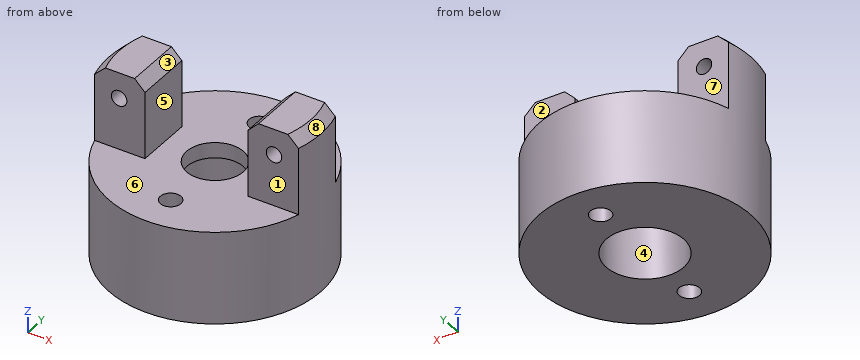
from build123d import *

# Parameters (mm, degrees)
SKETCH_1_R          = 20.5
EXTRUDE_1_DEPTH     = 33
CUT_EXTRUDE_1_DEPTH = 15
SKETCH_3_R          = 5
SKETCH_3_R_2        = 2
CUT_EXTRUDE_2_DEPTH = 35.124771062
CHAMFER_1_SIZE      = 2
SKETCH_4_R          = 1.5
CUT_EXTRUDE_3_DEPTH = 15
SKETCH_6_R          = 5.5
CUT_EXTRUDE_4_DEPTH = 35.124771062
SKETCH_9_R          = 7.5
CUT_EXTRUDE_7_DEPTH = 15


with BuildPart() as part:
    # Эскиз1 → Вытянуть1 (new body)
    with BuildSketch(Plane.XY):
        Circle(SKETCH_1_R)
    extrude(amount=EXTRUDE_1_DEPTH)

    # Эскиз2 → Вырез-Вытянуть1 (cut)
    with BuildSketch(Plane.XY.offset(33)):
        Polygon((10, 5.5), (24.402362137, 5.5), (24.402362137, 27.166317261), (-29.05675736, 27.166317261), (-29.05675736, 5.5), (-10, 5.5), (-10, -5.5), (-25.152295152, -5.5), (-25.152295152, -27.51572327), (25.537931669, -27.51572327), (25.537931669, -5.5), (10, -5.5), align=None)
    extrude(amount=-CUT_EXTRUDE_1_DEPTH, mode=Mode.SUBTRACT)

    # Эскиз3 → Вырез-Вытянуть2 (cut, through all)
    with BuildSketch(Plane.XY.offset(18)):
        Circle(SKETCH_3_R)
        with Locations((0, 13.25)):
            Circle(SKETCH_3_R_2)
        with Locations((0, -13.25)):
            Circle(SKETCH_3_R_2)
    extrude(amount=-CUT_EXTRUDE_2_DEPTH, mode=Mode.SUBTRACT)

    # Фаска1
    chamfer_1_edges = [part.edges().sort_by_distance(p)[0] for p in [
        (-10, 0, 33),
        (10, 0, 33),
        (-20.5, 0, 33),
        (20.311235339, -2.775557422, 33),
    ]]
    chamfer(chamfer_1_edges, length=CHAMFER_1_SIZE)

    # Эскиз4 → Вырез-Вытянуть3 (cut)
    with BuildSketch(Plane.XZ.offset(5.5)):
        with Locations((-15, 28)):
            Circle(SKETCH_4_R)
        with Locations((15, 28)):
            Circle(SKETCH_4_R)
    extrude(amount=-CUT_EXTRUDE_3_DEPTH, mode=Mode.SUBTRACT)

    # Эскиз6 → Вырез-Вытянуть4 (cut, through all)
    with BuildSketch(Plane.XY.offset(18)):
        Circle(SKETCH_6_R)
    extrude(amount=-CUT_EXTRUDE_4_DEPTH, mode=Mode.SUBTRACT)

    # Эскиз9 → Вырез-Вытянуть7 (cut)
    with BuildSketch(Plane(origin=(0, 0, 0), x_dir=(-1, 0, 0), z_dir=(0, 0, -1))):
        Circle(SKETCH_9_R)
    extrude(amount=-CUT_EXTRUDE_7_DEPTH, mode=Mode.SUBTRACT)


solid = part.part
Input: part model. Units: mm. Frame: model coordinates. Face numbers are marked on the shaded views. A direction names the side the tool comes from. Give positions to 0.01 mm unless a question says otherwise; leave off trailing zeros. Loops run counter-clockwise (first coordinate to the right, second up) from the corner with the lowest first, then second, coordinate; pieces in that order, holes last. Notation, with made-up numbers: (-39, -36) -> (16, -36) arc R23 ccw to (16, -15) -> close; hole circle Ø7 at (-32.75, -4). An arc over 180 degrees is marked (long way). Answer as a JSON object with one key per item and string values. Group by question number.
Item 1: Pin query (flat end, axial travel): P1, Ø5, axis at x = -10, y = 13, coming from the +Z side; P2, Ø8, axis at x = 14, z = 23.5, coming from the +Y side; P3, Ø5, axis at x = 16, z = 24, coming from the -Y side. Return the tip coordinate at first contact, or that it passes through.
Item 2: Pull-direction query (X, two-part tool) for the marked faces 5, 6, 7 and 8; classes: released by +X, released by -X, zero draft, split by the parting line, or undercut.
Item 3: Reachability of the marked faces 1, 2, 3 and 4 from +Z, -Z, +X, -X, +Y, -Y: full face, straight path, thin tool, end or side. Return the list, or none.
Item 4: Cut plane B-B, the plane z = 19. Return the cut outline in (x, y).
Item 5: Cut plane C-C, the plane x = -4.5. Return the cut outline in (y, z), and give its area (3 significant figures).
Item 6: Cut plane A-A, the plane y = 0. Return the cut outline in (x, z).
Item 7: Cut plane D-D, the plane z = 28. Return the cut outline in (x, y).
Item 8: Line query: probe 1 along Y at (x, z) = (0, 10.5); probe 2 along Z at (x, y) = (-10.5, 10.5); probe 3 along X at (y, z) = (13, 8). Output: solid intervals per line, ascending.
Checks:
{
 "1": {"P1": "stops at z = 18", "P2": "stops at y = 5.5", "P3": "stops at y = -5.5"},
 "2": {"face 5": "undercut", "face 6": "undercut", "face 7": "zero draft", "face 8": "released by +X"},
 "3": {"face 1": "+Z, +X, -X, -Y", "face 2": "+Z, +X, -X, +Y", "face 3": "+Z, +Y, -Y", "face 4": "-Z"},
 "4": {"outline": "(-19.75, -5.5) -> (-10, -5.5) -> (-10, 5.5) -> (-19.75, 5.5) arc R20.5 ccw to start; (10, -5.5) -> (19.75, -5.5) arc R20.5 ccw to (19.75, 5.5) -> (10, 5.5) -> close"},
 "5": {"outline": "(-20, 0) -> (-6, 0) -> (-6, 15) -> (-3.16, 15) -> (-3.16, 18) -> (-20, 18) -> close; (3.16, 15) -> (6, 15) -> (6, 0) -> (20, 0) -> (20, 18) -> (3.16, 18) -> close", "area": "521 mm²"},
 "6": {"outline": "(-20.5, 0) -> (-7.5, 0) -> (-7.5, 15) -> (-5.5, 15) -> (-5.5, 18) -> (-10, 18) -> (-10, 31) -> (-12, 33) -> (-18.5, 33) -> (-20.5, 31) -> close; (5.5, 15) -> (7.5, 15) -> (7.5, 0) -> (20.5, 0) -> (20.5, 31) -> (18.5, 33) -> (12, 33) -> (10, 31) -> (10, 18) -> (5.5, 18) -> close; hole circle Ø3 at (-15, 28); hole circle Ø3 at (15, 28)"},
 "7": {"outline": "(-19.75, -5.5) -> (-16.5, -5.5) -> (-16.5, 5.5) -> (-19.75, 5.5) arc R20.5 ccw to start; (-13.5, -5.5) -> (-10, -5.5) -> (-10, 5.5) -> (-13.5, 5.5) -> close; (10, -5.5) -> (13.5, -5.5) -> (13.5, 5.5) -> (10, 5.5) -> close; (16.5, -5.5) -> (19.75, -5.5) arc R20.5 ccw to (19.75, 5.5) -> (16.5, 5.5) -> close"},
 "8": {"probe 1": "y = -20.5 to -15.25, -11.25 to -7.5, 7.5 to 11.25, 15.25 to 20.5", "probe 2": "z = 0 to 18", "probe 3": "x = -15.85 to -1.98, 1.98 to 15.85"}
}
